```python
from build123d import *

# Parameters (mm, degrees)
CROQUIS1_W              = 50
CROQUIS1_H              = 105
SALIENTE_EXTRUIR1_DEPTH = 6
CROQUIS2_R              = 3.6
CROQUIS2_R_2            = 2.55
CORTAR_EXTRUIR2_DEPTH   = 7
CROQUIS4_R              = 6
CROQUIS4_R_2            = 5.05
CORTAR_EXTRUIR3_DEPTH   = 2
CROQUIS5_R              = 1.55
CROQUIS5_W              = 6
CROQUIS5_H              = 4.2
CORTAR_EXTRUIR4_DEPTH   = 7
CORTAR_EXTRUIR6_DEPTH   = 7
CROQUIS14_R             = 3
CORTAR_EXTRUIR9_DEPTH   = 2.5
CROQUIS16_R             = 15
CORTAR_EXTRUIR10_DEPTH  = 7
CROQUIS17_R             = 1.55
CROQUIS17_W             = 4
CROQUIS17_H             = 6
CORTAR_EXTRUIR11_DEPTH  = 7
REDONDEO1_R             = 5
CORTAR_EXTRUIR12_DEPTH  = 7


with BuildPart() as part:
    # Croquis1 → Saliente-Extruir1 (new body)
    with BuildSketch(Plane(origin=(0, 0, 0), x_dir=(1, 0, 0), z_dir=(0, 1, 0))):
        Rectangle(CROQUIS1_W, CROQUIS1_H)
    extrude(amount=SALIENTE_EXTRUIR1_DEPTH)

    # Croquis2 → Cortar-Extruir2 (cut, through all)
    with BuildSketch(Plane(origin=(0, 6, 0), x_dir=(1, 0, 0), z_dir=(0, 1, 0))):
        with Locations((-15, 36.45)):
            Circle(CROQUIS2_R)
        with Locations((15, 36.45)):
            Circle(CROQUIS2_R)
        with Locations((15, -15.45)):
            Circle(CROQUIS2_R_2)
        with Locations((-15, -15.45)):
            Circle(CROQUIS2_R_2)
    extrude(amount=-CORTAR_EXTRUIR2_DEPTH, mode=Mode.SUBTRACT)

    # Croquis4 → Cortar-Extruir3 (cut)
    with BuildSketch(Plane.XZ):
        with Locations((15, -36.45)):
            Circle(CROQUIS4_R)
        with Locations((-15, -36.45)):
            Circle(CROQUIS4_R)
        with Locations((-15, 15.45)):
            Circle(CROQUIS4_R_2)
        with Locations((15, 15.45)):
            Circle(CROQUIS4_R_2)
    extrude(amount=-CORTAR_EXTRUIR3_DEPTH, mode=Mode.SUBTRACT)

    # Croquis5 → Cortar-Extruir4 (cut, through all)
    with BuildSketch(Plane(origin=(0, 6, 0), x_dir=(1, 0, 0), z_dir=(0, 1, 0))):
        with Locations((0, 47.5)):
            Circle(CROQUIS5_R)
        with Locations((-11, 47.5)):
            Rectangle(CROQUIS5_W, CROQUIS5_H)
        with Locations((11, 47.5)):
            Rectangle(CROQUIS5_W, CROQUIS5_H)
    cortar_extruir4 = extrude(amount=-CORTAR_EXTRUIR4_DEPTH, mode=Mode.SUBTRACT)

    # Croquis8 → Cortar-Extruir6 (cut, through all)
    with BuildSketch(Plane(origin=(0, 6, 0), x_dir=(1, 0, 0), z_dir=(0, 1, 0))):
        with BuildLine():
            Line((-11.878679656, 49.6), (-10.121320344, 49.6))
            ThreePointArc((-10.121320344, 49.6), (-8.010608171, 49.610503119), (-7.979099854, 47.5))
            ThreePointArc((-7.979099854, 47.5), (-8.010608171, 45.389496881), (-10.121320344, 45.4))
            Line((-10.121320344, 45.4), (-11.878679656, 45.4))
            ThreePointArc((-11.878679656, 45.4), (-13.989391829, 45.389496881), (-14.020900146, 47.5))
            ThreePointArc((-14.020900146, 47.5), (-13.989391829, 49.610503119), (-11.878679656, 49.6))
        make_face()
        with BuildLine():
            Line((10.121320344, 45.4), (11.878679656, 45.4))
            ThreePointArc((11.878679656, 45.4), (13.989391829, 45.389496881), (14.020900146, 47.5))
            ThreePointArc((14.020900146, 47.5), (13.989391829, 49.610503119), (11.878679656, 49.6))
            Line((11.878679656, 49.6), (10.121320344, 49.6))
            ThreePointArc((10.121320344, 49.6), (8.010608171, 49.610503119), (7.979099854, 47.5))
            ThreePointArc((7.979099854, 47.5), (8.010608171, 45.389496881), (10.121320344, 45.4))
        make_face()
    cortar_extruir6 = extrude(amount=-CORTAR_EXTRUIR6_DEPTH, mode=Mode.SUBTRACT)

    # Simetría1: Cortar-Extruir4, Cortar-Extruir6 across plane
    add(cortar_extruir4.mirror(Plane.XY.offset(-30)), mode=Mode.SUBTRACT)
    add(cortar_extruir6.mirror(Plane.XY.offset(-30)), mode=Mode.SUBTRACT)

    # Croquis14 → Cortar-Extruir9 (cut)
    with BuildSketch(Plane(origin=(0, 6, 0), x_dir=(1, 0, 0), z_dir=(0, 1, 0))):
        with Locations((0, 12.5)):
            Circle(CROQUIS14_R)
    extrude(amount=-CORTAR_EXTRUIR9_DEPTH, mode=Mode.SUBTRACT)

    # Croquis16 → Cortar-Extruir10 (cut, through all)
    with BuildSketch(Plane.XZ):
        with Locations((0, 35.5)):
            Circle(CROQUIS16_R)
    extrude(amount=-CORTAR_EXTRUIR10_DEPTH, mode=Mode.SUBTRACT)

    # Croquis17 → Cortar-Extruir11 (cut, through all)
    with BuildSketch(Plane(origin=(0, 6, 0), x_dir=(1, 0, 0), z_dir=(0, 1, 0))):
        with Locations((21, -35.5)):
            Circle(CROQUIS17_R)
        with Locations((-21, -35.5)):
            Circle(CROQUIS17_R)
        with Locations((-21, -43.5)):
            Rectangle(CROQUIS17_W, CROQUIS17_H)
        with Locations((21, -43.5)):
            Rectangle(CROQUIS17_W, CROQUIS17_H)
        with Locations((21, -27.5)):
            Rectangle(CROQUIS17_W, CROQUIS17_H)
        with Locations((-21, -27.5)):
            Rectangle(CROQUIS17_W, CROQUIS17_H)
    extrude(amount=-CORTAR_EXTRUIR11_DEPTH, mode=Mode.SUBTRACT)

    # Redondeo1
    redondeo1_edges = [part.edges().sort_by_distance(p)[0] for p in [
        (25, 3, 52.5),
        (-25, 3, 52.5),
        (-25, 3, -52.5),
        (25, 3, -52.5),
    ]]
    fillet(redondeo1_edges, radius=REDONDEO1_R)

    # Croquis18 → Cortar-Extruir12 (cut, through all)
    with BuildSketch(Plane(origin=(0, 6, 0), x_dir=(1, 0, 0), z_dir=(0, 1, 0))):
        with BuildLine():
            ThreePointArc((-21, -24.391198464), (-23.439339828, -25.560660172), (-21, -26.73012188))
            ThreePointArc((-21, -26.73012188), (-18.560660172, -25.560660172), (-21, -24.391198464))
        make_face()
        with BuildLine():
            ThreePointArc((-21, -30.608801536), (-23.439339828, -29.439339828), (-21, -28.26987812))
            ThreePointArc((-21, -28.26987812), (-18.560660172, -29.439339828), (-21, -30.608801536))
        make_face()
        with BuildLine():
            ThreePointArc((-21, -46.608801536), (-18.560660172, -45.439339828), (-21, -44.26987812))
            ThreePointArc((-21, -44.26987812), (-23.439339828, -45.439339828), (-21, -46.608801536))
        make_face()
        with BuildLine():
            ThreePointArc((-21, -40.391198464), (-23.439339828, -41.560660172), (-21, -42.73012188))
            ThreePointArc((-21, -42.73012188), (-18.560660172, -41.560660172), (-21, -40.391198464))
        make_face()
        with BuildLine():
            ThreePointArc((21, -24.391198464), (18.560660172, -25.560660172), (21, -26.73012188))
            ThreePointArc((21, -26.73012188), (23.439339828, -25.560660172), (21, -24.391198464))
        make_face()
        with BuildLine():
            ThreePointArc((21, -30.608801536), (18.560660172, -29.439339828), (21, -28.26987812))
            ThreePointArc((21, -28.26987812), (23.439339828, -29.439339828), (21, -30.608801536))
        make_face()
        with BuildLine():
            ThreePointArc((21, -40.391198464), (18.560660172, -41.560660172), (21, -42.73012188))
            ThreePointArc((21, -42.73012188), (23.439339828, -41.560660172), (21, -40.391198464))
        make_face()
        with BuildLine():
            ThreePointArc((21, -46.608801536), (23.439339828, -45.439339828), (21, -44.26987812))
            ThreePointArc((21, -44.26987812), (18.560660172, -45.439339828), (21, -46.608801536))
        make_face()
    extrude(amount=-CORTAR_EXTRUIR12_DEPTH, mode=Mode.SUBTRACT)


solid = part.part
```
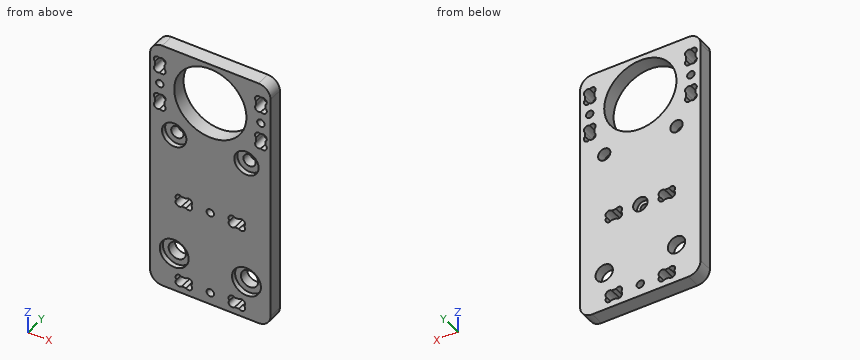
For this review, take the finished solid that the model builds, in its own axes (mm). Give positions to 0.01 mm unless a question says otherwise; leave off trailing zeros. Write each loop counter-clockwise with the first axis right and the second up, starting at its lowest first coordinate (ties: lowest second). Pieces come first, ordered by that corner, then holes. Notation, with made-up numbers: M 15.5,-24 L 45.5,-24 A11 ccw 45.5,-20 Z; hole C 85.25,-7.5 d9. An arc over 180 degrees is marked long. Answer as a JSON object with one key per item and string values. Group by question number.
Item 1: Consider section D-D on x = -16. Write out the cut boundary in (y, z).
Item 2: Consider section A-A on x = 0. Write out the cut boundary in (y, z).
Item 3: Consider section B-B on z = 35.5. Write out the cut boundary in (x, y).
Item 4: For probe 1 along Z at (x, y) = (0, 2.7); probe 2 along Z at (x, y) = (9, 2.8); probe 3 along Z at (x, y) = (13, 2.35), list the stretches that pass through material, from the lowest coordinate up. Write a range as [from, to].
Item 5: Consider section C-C on z = 15.45. Write out the cut boundary in (x, y), plus the area to 3 significant figures.
Item 6: For pin 1 Ø2.5 at (x, z) = (0, -47.5) entering from -Y; pin 2 Ø6 at (x, z) = (17, -38) entering from -Y, all flat-tipped, find the tip position at first contact; note any pin that passes through.
Check result:
{
 "1": {"outline": "M 0,-52.5 L 6,-52.5 L 6,-39.91 L 2,-39.91 L 2,-42.37 L 0,-42.37 Z; M 0,-30.53 L 2,-30.53 L 2,-32.99 L 6,-32.99 L 6,13.1 L 2,13.1 L 2,10.5 L 0,10.5 Z; M 0,20.4 L 2,20.4 L 2,17.8 L 6,17.8 L 6,52.5 L 0,52.5 Z"},
 "2": {"outline": "M 0,-52.5 L 6,-52.5 L 6,-49.05 L 0,-49.05 Z; M 0,-45.95 L 6,-45.95 L 6,-15.5 L 3.5,-15.5 L 3.5,-14.05 L 0,-14.05 Z; M 0,-10.95 L 3.5,-10.95 L 3.5,-9.5 L 6,-9.5 L 6,20.5 L 0,20.5 Z; M 0,50.5 L 6,50.5 L 6,52.5 L 0,52.5 Z"},
 "3": {"outline": "M -25,0 L -22.55,0 L -22.55,6 L -25,6 Z; M -19.45,0 L -15,0 L -15,6 L -19.45,6 Z; M 15,0 L 19.45,0 L 19.45,6 L 15,6 Z; M 22.55,0 L 25,0 L 25,6 L 22.55,6 Z"},
 "4": {"probe 1": "z = [-52.5, -49.05], [-45.95, -14.05], [-10.95, 20.5], [50.5, 52.5]", "probe 2": "z = [-52.5, -50.04], [-44.96, -15.04], [-9.96, 23.5], [47.5, 52.5]", "probe 3": "z = [-52.5, -50.04], [-44.96, -39.44], [-33.46, -15.04], [-9.96, 13.87], [17.03, 28.02], [42.98, 52.5]"},
 "5": {"outline": "M -25,0 L -20.05,0 L -20.05,2 L -17.55,2 L -17.55,6 L -25,6 Z; M -12.45,2 L -9.95,2 L -9.95,0 L 9.95,0 L 9.95,2 L 12.45,2 L 12.45,6 L -12.45,6 Z; M 17.55,2 L 20.05,2 L 20.05,0 L 25,0 L 25,6 L 17.55,6 Z", "area": "219 mm^2"},
 "6": {"pin 1": "passes through", "pin 2": "stops at y = 2"}
}
